Autodesk Inventor part; units mm, degrees
ref_plane "YZ Plane" through (0, 0, 0) normal (1, 0, 0) x (0, 1, 0)
ref_plane "XZ Plane" through (0, 0, 0) normal (0, 1, 0) x (-1, 0, 0)
ref_plane "XY Plane" through (0, 0, 0) normal (0, 0, 1) x (1, 0, 0)
sketch "Sketch1" plane through (0, 0, 0) normal (0, 0, 1) x (1, 0, 0)
  line L0 (0, 0) -> (40, 0)
  line L1 (40, 0) -> (40, 30)
  line L2 (40, 30) -> (0, 30)
  line L3 (0, 30) -> (0, 0)
  line L4 (40, 20) -> (155, 20)
  line L5 (155, 20) -> (155, 10)
  line L6 (155, 10) -> (40, 10)
  line L7 (40, 10) -> (40, 20)
  point P0 (40, 10)
  dimension "d0" = 30
  dimension "d1" = 40
  dimension "d2" = 10
  dimension "d3" = 115
  dimension "d4" = 10
extrude "Extrusion1" add sketch "Sketch1" along normal blind 10
sketch "Sketch2" plane through (40, 20, 0) normal (0, 1, 0) x (1, 0, 0)
  circle A0 centre (110, -5) radius 2.5
  circle A1 centre (10, -5) radius 2.5
  line L0 (115, 0) -> (115, -10)
  line L1 (115, -10) -> (0, -10)
  line L2 (0, 0) -> (0, -10)
  line L3 (110, -7.5) -> (10, -7.5)
  line L4 (10, -7.5) -> (10, -2.5)
  line L5 (10, -2.5) -> (110, -2.5)
  line L6 (110, -2.5) -> (110, -7.5)
  point P0 (-40, 0)
  point P1 (110, -2.5)
  point P2 (10, -7.5)
  point P3 (10, -7.5)
  dimension "d8" = 5
  dimension "d12" = 5
  dimension "d9" = 5
  dimension "d10" = 5
  dimension "d11" = 10
  dimension "d14" = 2.5
  dimension "d22" = 100
  dimension "d23" = 5
extrude "Extrusion2" cut sketch "Sketch2" against normal blind 10
sketch "Sketch3" plane through (0, 30, 0) normal (0, 1, 0) x (1, 0, 0)
  circle A0 centre (5, -5) radius 2.5
  line L0 (0, 0) -> (0, -10)
  line L1 (40, 0) -> (0, 0)
  dimension "d17" = 5
  dimension "d18" = 5
  dimension "d19" = 5
extrude "Extrusion3" cut sketch "Sketch3" against normal blind 30
properties part number "Top Piece"
Read the model definition and answer for the solid it produces. Units are mm, in the model's axes. A direction names the side the tool comes from. Round coordinates to 2 decimals unless told otherwise and drop trailing zeros. Loops run counter-clockwise (first coordinate to the right, second up) from the corner with the lowest first, then second, coordinate; pieces in that order, holes last.
Q1. Determine the mould class of faces 1 (the face through (7.385, 15.21, 4.249)), 2 (the face through (97, 20, 2)), 3 (the face through (40, 25, 5)) for opening direction X: released by +X, released by -X, zero draft, split by the parting line, or undercut.
Q2. Section D-D on x = 5 is taken. Write down the section's boundary in (y, z), and give its area (3 significant figures).
Q3. Which of the six approach directions +Z, -Z, +X, -X, +Y, -Y give full straight-line access (tool end or side, diameter ignored) to faces 4 (the face through (40, 5, 5)), 5 (the face through (20, 30, 5)), 6 (the face through (152.5, 15.1, 5.1))?
Q4. Section C-C on y = 7.75 is taken. Write down the section's boundary in (x, z).
Q5. Consider probe 1 along Z at (x, y) = (148, 12.25); probe 2 along X at (y, z) = (10.5, 5); probe 3 along X at (y, z) = (9.75, 8). Determine where each line is inside the solid, lowest interval first.
Q6. Each of these flat-tipped pins is pushed along its axis until it touches: pin 1 (6 mm diameter, centred on x = 49, y = 21.5, fed in from -Z); pin 2 (3 mm diameter, centred on y = 23.5, z = 7, fed in from +X); pin 3 (4 mm diameter, centred on x = 132, z = 4, fed in from +Y). Where does it stop, or does it pass through?
Q7. Section A-A on x = 121.5 is taken. Write down the section's boundary in (y, z).
Q8. Section B-B on z = 5 is taken. Write down the section's boundary in (x, y).
Output:
1. face 1: undercut
1. face 2: zero draft
1. face 3: released by +X
2. outline: (0, 0) - (30, 0) - (30, 2.5) - (0, 2.5) - close; (0, 7.5) - (30, 7.5) - (30, 10) - (0, 10) - close
2. area: 150 mm2
3. face 4: +Z, -Z, +X, -Y
3. face 5: +Z, -Z, +X, -X, +Y
3. face 6: +Y, -Y
4. outline: (0, 0) - (40, 0) - (40, 10) - (0, 10) - close; hole circle Ø5 at (5, 5)
5. probe 1: z = 0 to 2.5, 7.5 to 10
5. probe 2: x = 0 to 2.5, 7.5 to 47.5, 152.5 to 155
5. probe 3: x = 0 to 40
6. pin 1: stops at z = 0
6. pin 2: stops at x = 40
6. pin 3: stops at y = 20
7. outline: (10, 0) - (20, 0) - (20, 2.5) - (10, 2.5) - close; (10, 7.5) - (20, 7.5) - (20, 10) - (10, 10) - close
8. outline: (0, 0) - (2.5, 0) - (2.5, 30) - (0, 30) - close; (7.5, 0) - (40, 0) - (40, 10) - (47.5, 10) - (47.5, 20) - (40, 20) - (40, 30) - (7.5, 30) - close; (152.5, 10) - (155, 10) - (155, 20) - (152.5, 20) - close
